Design review of the part built by this model. Coordinates are the model's own, in mm. Coordinates: 2 decimals unless noted, no trailing zeros. Write each loop counter-clockwise with the first axis right and the second up, starting at its lowest first coordinate (ties: lowest second). Pieces come first, ordered by that corner, then holes.
Q1. Take a section at D-D (x = 3). Give the boundary of the cut face in (y, z), and give its area (3 significant figures).
Q2. Insertion check: pin 1 (1 mm diameter, centred on x = 15, y = 16, fed in from -Z); pin 2 (10 mm diameter, centred on y = 0, z = 25.4, fed in from +X); pin 3 (2 mm diameter, centred on y = 17, z = 45.5, fed in from -X). Each pin has a flat end and moves straight along its axis. Give the tip position at first contact, or say it passes through.
Q3. For probe 1 along Z at (x, y) = (19.5, 0); probe 2 along Y at (x, z) = (20, 25); probe 3 along Y at (x, z) = (19, 32), list the stretches that pass through material, from the lowest coordinate up.
Q4. Mouldability with a two-part tool opening along Y and no side actions: class faces 1 (the flat face through (0, 25.4, 26)), 2 (the flat face through (25.651, -6, 31)), 3 (the cylindrical face through (13.129, 2.93, 19.766)), 4 (the flat face through (0.251, 0, 25)) as pulls with the +Y half, pulls with the -Y half, needs draft (parallel to the pull), parting line crosses it, or undercut.
Q5. Take a section at A-A (x = 17). Give the boundary of the cut face in (y, z), and give its area (3 significant figures).
Q6. Take a section at C-C (y = -19). Give the boundary of the cut face in (x, z).
Q7. Take a section at B-B (z = 36). Give the boundary of the cut face in (x, y), and give its area (3 significant figures).
```python
from build123d import *

# Parameters (mm, degrees)
F0_W      = 50.8
F0_H      = 50.8
F1_DEPTH  = 25.4
F9_W      = 81.569908
F9_H      = 70.63064
F10_DEPTH = 29.3
F12_R     = 89.535531
F13_DEPTH = 25
F15_R     = 39.569466
F16_DEPTH = 41
F18_W     = 58.592394
F18_H     = 71.147578
F19_DEPTH = 100
F21_W     = 80.173537
F21_H     = 55.645675
F22_DEPTH = 42.7
F24_W     = 87.651257
F24_H     = 68.795107
F25_DEPTH = 25
F27_W     = 100.011413
F27_H     = 117.008079
F28_DEPTH = 25
F30_W     = 0.249144
F30_H     = 2.697075
F31_DEPTH = 48.9
F32_R     = 6.35
F33_DEPTH = 25.4


with BuildPart() as f1:
    # F0 (on Front) → F1 (new body, symmetric)
    with BuildSketch(Plane.XZ):
        with Locations((0.251064, 25.4)):
            Rectangle(F0_W, F0_H)
    extrude(amount=F1_DEPTH, both=True)

    # F9 (on face) → F10 (cut)
    with BuildSketch(Plane(origin=(-8.382979, 8.382979, -8.382979), x_dir=(-0.408248, -0.816497, -0.408248), z_dir=(-0.57735, 0.57735, -0.57735))):
        with Locations((-10.190026, 10.921631)):
            Rectangle(F9_W, F9_H)
    extrude(amount=F10_DEPTH, mode=Mode.SUBTRACT)

    # F12 (on face) → F13 (cut)
    with BuildSketch(Plane(origin=(8.550355, 8.550355, -8.550355), x_dir=(0.408248, -0.816497, -0.408248), z_dir=(-0.57735, -0.57735, 0.57735))):
        with Locations((-35.490789, 68.001591)):
            Circle(F12_R)
    extrude(amount=-F13_DEPTH, mode=Mode.SUBTRACT)

    # F15 (on face) → F16 (cut)
    with BuildSketch(Plane(origin=(25.483688, 25.483688, 25.483688), x_dir=(0.408248, -0.816497, 0.408248), z_dir=(-0.57735, -0.57735, -0.57735))):
        with Locations((9.887295, 17.477341)):
            Circle(F15_R)
    extrude(amount=-F16_DEPTH, mode=Mode.SUBTRACT)

    # F18 (on face) → F19 (cut)
    with BuildSketch(Plane(origin=(-25.484761, 25.230394, 25.230394), x_dir=(-0.408912, -0.817865, 0.404831), z_dir=(-0.581211, 0.57541, 0.57541))):
        with Locations((4.633598, 13.250503)):
            Rectangle(F18_W, F18_H)
    extrude(amount=F19_DEPTH, mode=Mode.SUBTRACT)

    # F21 (on face) → F22 (cut)
    with BuildSketch(Plane(origin=(-25.316312, -25.316312, 25.316312), x_dir=(0.816497, -0.408248, 0.408248), z_dir=(-0.57735, -0.57735, 0.57735))):
        with Locations((7.817443, 21.68025)):
            Rectangle(F21_W, F21_H)
    extrude(amount=F22_DEPTH, mode=Mode.SUBTRACT)

    # F24 (on face) → F25 (cut)
    with BuildSketch(Plane(origin=(-8.494105, -8.410968, -8.410968), x_dir=(-0.408899, 0.817838, -0.404897), z_dir=(0.581136, 0.575448, 0.575448))):
        with Locations((-14.611577, 10.17838)):
            Rectangle(F24_W, F24_H)
    extrude(amount=-F25_DEPTH, mode=Mode.SUBTRACT)

    # F27 (on face) → F28 (cut)
    with BuildSketch(Plane(origin=(8.410968, -8.410968, -8.494105), x_dir=(0.817838, 0.404897, 0.408899), z_dir=(-0.575448, 0.575448, 0.581136))):
        with Locations((1.137109, -4.921732)):
            Rectangle(F27_W, F27_H)
    extrude(amount=-F28_DEPTH, mode=Mode.SUBTRACT)

    # F30 (on face) → F31 (cut)
    with BuildSketch(Plane(origin=(25.315773, -25.566005, 25.566005), x_dir=(0.81916, 0.405571, -0.405571), z_dir=(0.573565, -0.579234, 0.579234))):
        Polygon((-45.404907, 18.753311), (-67.2075, 18.753311), (-67.2075, -9.424486), (53.327814, -9.424486), (53.327814, 18.753311), (35.788387, 18.753311), align=None)
        with Locations((35.663815, 20.775202)):
            Rectangle(F30_W, F30_H)
        Polygon((-45.404907, 42.469528), (-45.404907, 18.753311), (35.788387, 18.753311), (35.788387, 19.426664), (35.539243, 19.426664), (35.539243, 22.123739), (35.788387, 22.123739), (35.788387, 42.469528), align=None)
    extrude(amount=F31_DEPTH, mode=Mode.SUBTRACT)

    # F32 (on face) → F33 (cut)
    with BuildSketch(Plane.YZ.offset(25.651064)):
        with Locations((0, 25.4)):
            Circle(F32_R)
    extrude(amount=-F33_DEPTH, mode=Mode.SUBTRACT)


solid = f1.part
```
Response:
1. outline: (-25.4, 2.97) - (-22.4, 0) - (22.65, 0) - (25.4, 2.75) - (25.4, 48.05) - (22.65, 50.8) - (-22.43, 50.8) - (-25.4, 47.83) - close; hole circle Ø12.7 at (0, 25.4)
1. area: 2,440 mm2
2. pin 1: stops at z = 4.64
2. pin 2: stops at x = 0.25
2. pin 3: stops at x = -14.97
3. probe 1: z = 0 to 19.05, 31.75 to 50.8
3. probe 2: y = -25.4 to -6.34, 6.34 to 25.4
3. probe 3: y = -25.39 to 25.4
4. face 1: pulls with the +Y half
4. face 2: needs draft
4. face 3: undercut
4. face 4: undercut
5. outline: (-25.4, 16.83) - (-8.4, 0) - (8.65, 0) - (25.4, 16.75) - (25.4, 34.05) - (8.65, 50.8) - (-8.57, 50.8) - (-25.4, 33.97) - close; hole circle Ø12.7 at (0, 25.4)
5. area: 1,890 mm2
6. outline: (-25.15, 19) - (-6.34, 0) - (6.4, 0) - (25.65, 19.06) - (25.65, 31.8) - (6.46, 50.8) - (-6.15, 50.8) - (-25.15, 31.8) - close
7. outline: (-25.15, -14.8) - (-14.55, -25.4) - (14.95, -25.4) - (25.65, -14.8) - (25.65, 14.8) - (15.05, 25.4) - (-14.65, 25.4) - (-25.15, 14.8) - close
7. area: 2,360 mm2
